The drawing under review shows one solid part. Ordinate dimensions are in mm from its lowest x, y, z. Coordinates: 2 decimals unless noted, no trailing zeros. Write each loop counter-clockwise with the first axis right and the second up, starting at its lowest first coordinate (ties: lowest second). Pieces come first, ordered by that corner, then holes.
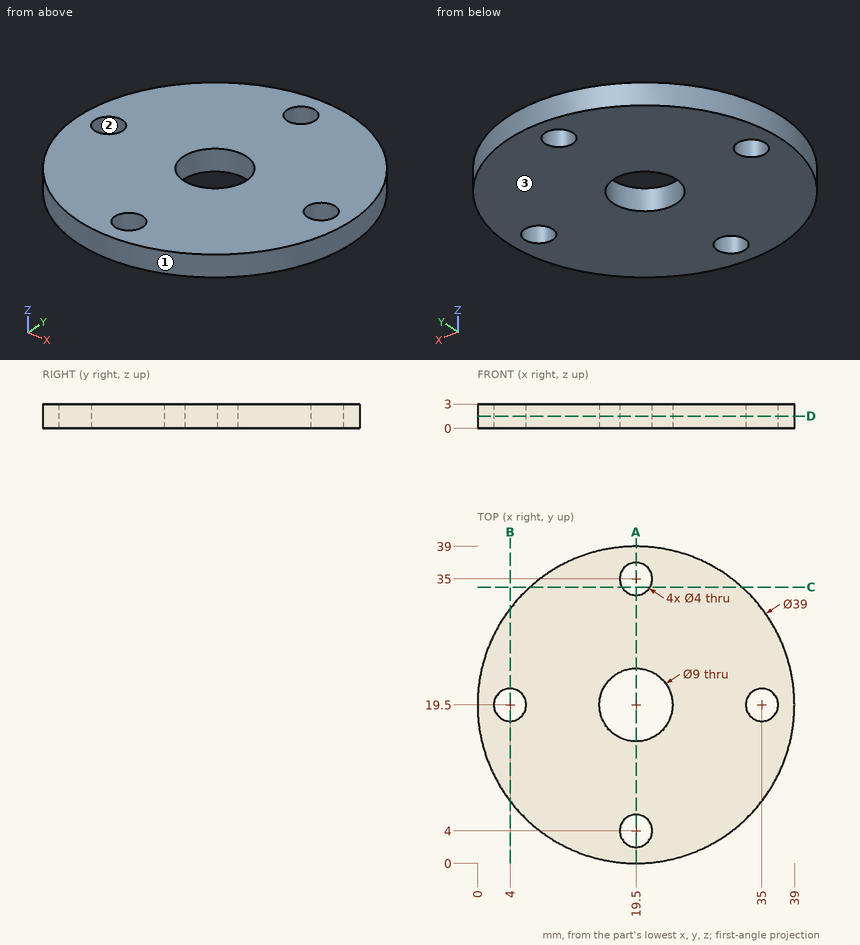
1) Consider section C-C (y = 34). Give the boundary of the cut face in (x, z), then the cut area to 3 significant figures.
2) Consider section D-D (z = 1.5). Give the boundary of the cut face in (x, y), then the cut area to 3 significant figures.
3) The part is to be moulded in two halves that separate along Y. For the marked faces 1, 2 and 3, say which applies: pulls with the +Y half, pulls with the -Y half, needs draft (parallel to the pull), parting line crosses it, or undercut.
4) Clearance check with a flat-ended pin moving along its axis: P1, Ø1, axis at x = 19.5, z = 1, coming from the +Y side. State where the tip first meets the part, or that it passes through.
5) Consider section B-B (x = 4). Give the boundary of the cut face in (y, z).
6) Consider section A-A (x = 19.5). Give the boundary of the cut face in (y, z).
7) For L1, parallel to Y at x = 19.5, z = 1.1; L2, parallel to Y at x = 36.5, z = 0.55; L3, parallel to Y at x = 35, z = 0.8, list the stretches that pass through material, from the lowest coordinate up.
Results:
1. outline: (6.46, 0) - (17.77, 0) - (17.77, 3) - (6.46, 3) - close; (21.23, 0) - (32.54, 0) - (32.54, 3) - (21.23, 3) - close
1. area: 67.8 mm2
2. outline: circle Ø39 at (19.5, 19.5); hole circle Ø4 at (4, 19.5); hole circle Ø9 at (19.5, 19.5); hole circle Ø4 at (19.5, 4); hole circle Ø4 at (19.5, 35); hole circle Ø4 at (35, 19.5)
2. area: 1,080 mm2
3. face 1: parting line crosses it
3. face 2: undercut
3. face 3: needs draft
4. P1: stops at y = 39
5. outline: (7.67, 0) - (17.5, 0) - (17.5, 3) - (7.67, 3) - close; (21.5, 0) - (31.33, 0) - (31.33, 3) - (21.5, 3) - close
6. outline: (0, 0) - (2, 0) - (2, 3) - (0, 3) - close; (6, 0) - (15, 0) - (15, 3) - (6, 3) - close; (24, 0) - (33, 0) - (33, 3) - (24, 3) - close; (37, 0) - (39, 0) - (39, 3) - (37, 3) - close
7. L1: y = 0 to 2, 6 to 15, 24 to 33, 37 to 39
7. L2: y = 9.95 to 18.18, 20.82 to 29.05
7. L3: y = 7.67 to 17.5, 21.5 to 31.33
